Source: CAD feature listing. Evaluate the final solid. Frame: model axes, mm. Coordinates: 2 decimals unless noted, no trailing zeros. Order: outer loops, then holes, each group sorted by start corner. A loop starts at its lowest first (then second) coordinate and runs counter-clockwise, first axis right, second up. Notation, with made-up numbers: (-37, 56.5) -> (13, 56.5) arc R10 cw to (13, 65.5) -> close; hole circle Ø6 at (36, 52.5). An arc over 180 degrees is marked (long way). Put each result on its own line as item: value.
from build123d import *

# Parameters (mm, degrees)
SKETCH1_R           = 32.131
SKETCH1_R_2         = 2.032
BOSS_EXTRUDE1_DEPTH = 3.175
FILLET1_R           = 3.175


with BuildPart() as part:
    # Sketch1 → Boss-Extrude1 (new body)
    with BuildSketch(Plane(origin=(0, 0, 0), x_dir=(0, 0, -1), z_dir=(1, 0, 0))):
        with BuildLine():
            ThreePointArc((0.539277511, 38.477221063), (-34.317069018, 17.410517941), (-30.731600023, -23.159363571))
            ThreePointArc((-30.731600023, -23.159363571), (-32.777019562, -30.977797205), (-24.855674027, -29.376569399))
            ThreePointArc((-24.855674027, -29.376569399), (35.104868111, -15.761839864), (5.438477754, 38.094754504))
            ThreePointArc((5.438477754, 38.094754504), (3.677072288, 47.101407959), (0.539277511, 38.477221063))
        make_face()
        Circle(SKETCH1_R, mode=Mode.SUBTRACT)
        with Locations((3.306405321, 42.353354437)):
            Circle(SKETCH1_R_2, mode=Mode.SUBTRACT)
        with Locations((-29.315764749, -27.706540357)):
            Circle(SKETCH1_R_2, mode=Mode.SUBTRACT)
    extrude(amount=BOSS_EXTRUDE1_DEPTH)

    # Fillet1
    fillet1_edges = [part.edges().sort_by_distance(p)[0] for p in [
        (1.5875, -23.159363571, 30.731600023),
        (1.5875, 38.477221063, -0.539277511),
        (1.5875, 38.094754504, -5.438477754),
        (1.5875, -29.376569399, 24.855674027),
    ]]
    fillet(fillet1_edges, radius=FILLET1_R)


solid = part.part
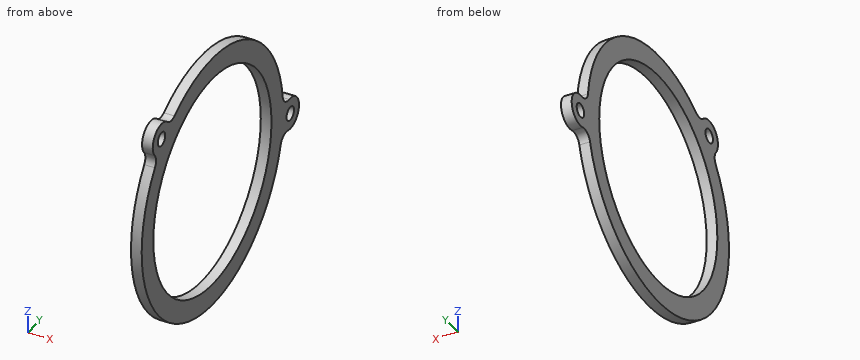
1. Cut plane A-A on y = 0. Output: boundary loops of the cut face in (x, z) (3 decimals).
Numbers:
outline: (0, -38.481) -> (3.175, -38.481) -> (3.175, -32.131) -> (0, -32.131) -> close; (0, 32.131) -> (3.175, 32.131) -> (3.175, 38.481) -> (0, 38.481) -> close
2. Cut plane B-B on z = 0. Output: boundary loops of the cut face in (x, y) (3 decimals).
Numbers:
outline: (0, -38.481) -> (3.175, -38.481) -> (3.175, -32.131) -> (0, -32.131) -> close; (0, 32.131) -> (3.175, 32.131) -> (3.175, 45.781) -> (0, 45.781) -> close
3. First-contact query: pin 1 (1.5 mm diameter, centred on x = 2, y = 34, fed in from +Z); pin 2 (1.5 mm diameter, centred on x = 2, z = -6.5, fed in from -Y). Flat tips, straight axial feed; report the tip coordinate or a pass-through.
Numbers:
pin 1: stops at z = 19.37
pin 2: stops at y = -38.05
4. Ray query, line 1 along Y through (x, z) = (1.8, 27.5); line 2 along Y through (x, z) = (1.4, -21); line 3 along Z through (x, y) = (2.65, -8.5). Return the intervals inside material, ascending.
Numbers:
line 1: y = -32.11 to -28.62, -26.79 to -16.62, 16.62 to 26.92
line 2: y = -32.25 to -24.32, 24.32 to 32.25
line 3: z = -37.53 to -30.99, 30.99 to 37.53
5. Cut plane C-C on x = 2.4. Count the separate pieces of the cut face and the enclosed holes in it, plus the area to 3 significant figures.
Numbers:
separate pieces: 1
enclosed holes: 3
area: 1,520 mm2
